```python
from build123d import *

# Parameters (mm, degrees)
CIRCLE034_R      = 2
EXTRUDE206_DEPTH = 2
CIRCLE_R         = 1
EXTRUDE086_DEPTH = 5
CIRCLE025_R      = 1
EXTRUDE088_DEPTH = 5
CIRCLE022_R      = 4
EXTRUDE160_DEPTH = 5
CIRCLE030_R      = 2.65
EXTRUDE173_DEPTH = 2
CIRCLE031_R      = 2.65
EXTRUDE174_DEPTH = 2
RECTANGLE045_W   = 19.3
RECTANGLE045_H   = 9.8
EXTRUDE085_DEPTH = 3.5
RECTANGLE043_W   = 29.4
RECTANGLE043_H   = 30
EXTRUDE083_DEPTH = 5
RECTANGLE044_W   = 1.5
RECTANGLE044_H   = 22.8
EXTRUDE095_DEPTH = 5


with BuildPart() as extrude206:
    # Circle034 → Extrude206 (new body)
    with BuildSketch(Plane(origin=(38.514674, -97.235972, -14.1), x_dir=(1, 0, 0), z_dir=(0, 0, 1))):
        Circle(CIRCLE034_R)
    extrude(amount=-EXTRUDE206_DEPTH)


with BuildPart() as extrude086:
    # Circle → Extrude086 (new body)
    with BuildSketch(Plane(origin=(27.579856, -94.349147, -14.1), x_dir=(1, 0, 0), z_dir=(0, 0, 1))):
        Circle(CIRCLE_R)
    extrude(amount=-EXTRUDE086_DEPTH)


with BuildPart() as extrude088:
    # Circle025 → Extrude088 (new body)
    with BuildSketch(Plane(origin=(27.579856, -115.349147, -14.1), x_dir=(1, 0, 0), z_dir=(0, 0, 1))):
        Circle(CIRCLE025_R)
    extrude(amount=-EXTRUDE088_DEPTH)


with BuildPart() as extrude160:
    # Circle022 → Extrude160 (new body)
    with BuildSketch(Plane(origin=(28.279856, -104.849147, -14.1), x_dir=(1, 0, 0), z_dir=(0, 0, 1))):
        Circle(CIRCLE022_R)
    extrude(amount=-EXTRUDE160_DEPTH)


with BuildPart() as extrude173:
    # Circle030 → Extrude173 (new body)
    with BuildSketch(Plane(origin=(27.579856, -94.349147, -19.1), x_dir=(1, 0, 0), z_dir=(0, 0, 1))):
        Circle(CIRCLE030_R)
    extrude(amount=EXTRUDE173_DEPTH)


with BuildPart() as extrude174:
    # Circle031 → Extrude174 (new body)
    with BuildSketch(Plane(origin=(27.579856, -115.349147, -19.1), x_dir=(1, 0, 0), z_dir=(0, 0, 1))):
        Circle(CIRCLE031_R)
    extrude(amount=EXTRUDE174_DEPTH)


with BuildPart() as extrude085:
    # Rectangle045 → Extrude085 (new body)
    with BuildSketch(Plane(origin=(22.779856, -109.749147, -14.1), x_dir=(1, 0, 0), z_dir=(0, 0, 1))):
        with Locations((9.65, 4.9)):
            Rectangle(RECTANGLE045_W, RECTANGLE045_H)
    extrude(amount=-EXTRUDE085_DEPTH)


with BuildPart() as cut107:
    # Rectangle043 → Extrude083 (new body)
    with BuildSketch(Plane(origin=(12.679856, -119.849147, -14.1), x_dir=(1, 0, 0), z_dir=(0, 0, 1))):
        with Locations((14.7, 15)):
            Rectangle(RECTANGLE043_W, RECTANGLE043_H)
    extrude(amount=-EXTRUDE083_DEPTH)

    # Cut027: cut Extrude085
    add(extrude085.part, mode=Mode.SUBTRACT)

    # Cut086: cut Extrude174
    add(extrude174.part, mode=Mode.SUBTRACT)

    # Cut087: cut Extrude173
    add(extrude173.part, mode=Mode.SUBTRACT)

    # Cut088: cut Extrude160
    add(extrude160.part, mode=Mode.SUBTRACT)

    # Cut089: cut Extrude088
    add(extrude088.part, mode=Mode.SUBTRACT)

    # Cut090: cut Extrude086
    add(extrude086.part, mode=Mode.SUBTRACT)

    # Cut107: cut Extrude206
    add(extrude206.part, mode=Mode.SUBTRACT)


with BuildPart() as fusion_lens_cover:
    # Rectangle044 → Extrude095 (new body)
    with BuildSketch(Plane(origin=(11.179856, -116.249147, -14.1), x_dir=(1, 0, 0), z_dir=(0, 0, 1))):
        with Locations((0.75, 11.4)):
            Rectangle(RECTANGLE044_W, RECTANGLE044_H)
    extrude(amount=-EXTRUDE095_DEPTH)

    # Fusion047: union Cut107
    add(cut107.part)


solid = fusion_lens_cover.part
```
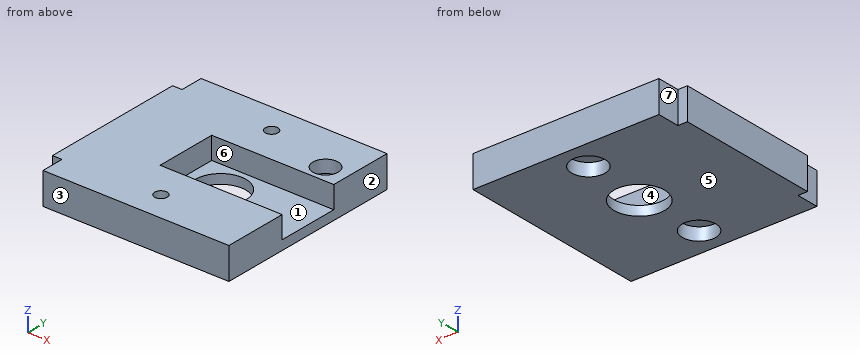
Geometry: final body of the model. Coordinates: model frame, mm. Face numbers are marked on the shaded views. A direction names the side the tool comes from. Round coordinates to 2 decimals unless told otherwise and drop trailing zeros. Order: outer loops, then holes, each group sorted by start corner. A loop starts at its lowest first (then second) coordinate and runs counter-clockwise, first axis right, second up. Notation, with made-up numbers: (52.5, 3) -> (108.5, 3) arc R24 cw to (108.5, 29) -> close; hole circle Ø8 at (25, 20). An arc over 180 degrees is marked (long way). Use one line per item in the form item = value.
(1) Section C-C on x = 37. Return loops of the section in (y, z), and give its area (3 significant figures).
Results list:
outline = (-119.85, -19.1) -> (-89.85, -19.1) -> (-89.85, -14.1) -> (-95.93, -14.1) -> (-95.93, -16.1) -> (-98.54, -16.1) -> (-98.54, -14.1) -> (-99.95, -14.1) -> (-99.95, -17.6) -> (-109.75, -17.6) -> (-109.75, -14.1) -> (-119.85, -14.1) -> close
area = 110 mm^2
(2) Draft query along Y for the marked faces 1, 2, 3 and 4. Return one class per face: pulls with the +Y half, pulls with the -Y half, needs draft (parallel to the pull), parting line crosses it, or undercut.
Results list:
face_1 = undercut
face_2 = needs draft
face_3 = pulls with the -Y half
face_4 = undercut
(3) Section D-D on y = -97.75. Return loops of the section in (x, z), and give its area (3 significant figures).
Results list:
outline = (11.18, -19.1) -> (42.08, -19.1) -> (42.08, -14.1) -> (40.45, -14.1) -> (40.45, -16.1) -> (36.58, -16.1) -> (36.58, -14.1) -> (11.18, -14.1) -> close
area = 147 mm^2
(4) Section B-B on z = -15.55. Return loops of the section in (x, y), and give its area (3 significant figures).
Results list:
outline = (11.18, -116.25) -> (12.68, -116.25) -> (12.68, -119.85) -> (42.08, -119.85) -> (42.08, -109.75) -> (22.78, -109.75) -> (22.78, -99.95) -> (42.08, -99.95) -> (42.08, -89.85) -> (12.68, -89.85) -> (12.68, -93.45) -> (11.18, -93.45) -> close; hole circle Ø2 at (27.58, -115.35); hole circle Ø2 at (27.58, -94.35); hole circle Ø4 at (38.51, -97.24)
area = 708 mm^2
(5) Section A-A on y = -101.25. Return loops of the section in (x, z).
Results list:
outline = (11.18, -19.1) -> (26.53, -19.1) -> (26.53, -17.6) -> (22.78, -17.6) -> (22.78, -14.1) -> (11.18, -14.1) -> close; (30.03, -19.1) -> (42.08, -19.1) -> (42.08, -17.6) -> (30.03, -17.6) -> close
(6) Access query for the marked faces 5, 6 and 7. Directions: +Z, -Z, +X, -X, +Y, -Y. A direction counts if a zero-diameter tool reaches every point of the face in a straight line with its end or side. Return the directions, or none.
Results list:
face_5 = -Z, +X, -X, +Y, -Y
face_6 = +Z, +X
face_7 = +Z, -Z, -X, +Y
(7) First-contact query: pin 1 Ø3 at (y, z) = (-106, -15.5) entering from +X; pin 2 Ø3 at (y, z) = (-118, -16.5) entering from -X; pin 3 Ø2.5 at (x, y) = (27.58, -115.35) entering from -Z. Flat tips, straight axial feed; report the tip coordinate or a pass-through.
Results list:
pin_1 = 22.78
pin_2 = 12.68
pin_3 = -17.1
(8) Ray query, probe 1 along Y at (x, z) = (33.5, -14.4); probe 2 along Y at (x, z) = (26.5, -17.5); probe 3 along Z at (x, y) = (28.5, -93). Return the intervals inside material, ascending. Write a range as [from, to].
Results list:
probe_1 = [-119.85, -109.75], [-99.95, -89.85]
probe_2 = [-119.85, -117.77], [-112.93, -109.75], [-99.95, -96.77], [-91.93, -89.85]
probe_3 = [-17.1, -14.1]
